```python
from build123d import *

# Parameters (mm, degrees)
SALIENTE_EXTRUIR1_DEPTH = 3
CORTAR_EXTRUIR1_DEPTH   = 10


with BuildPart() as part:
    # Croquis1 → Saliente-Extruir1 (new body)
    with BuildSketch(Plane(origin=(0, 0, 0), x_dir=(1, 0, 0), z_dir=(0, 1, 0))):
        Polygon((3, 35.5), (0, 35.5), (0, 47.5), (3, 47.5), (3, 59.5), (0, 59.5), (0, 71.5), (3, 71.5), (3, 80), (13.5, 80), (13.5, 83), (47.5, 83), (47.5, 80), (61, 80), (61, 71.5), (58, 71.5), (58, 59.5), (61, 59.5), (61, 47.5), (58, 47.5), (58, 35.5), (61, 35.5), (61, 23.5), (58, 23.5), (58, 11.5), (61, 11.5), (61, 3), (47.5, 3), (47.5, 0), (13.5, 0), (13.5, 3), (3, 3), (3, 11.5), (0, 11.5), (0, 23.5), (3, 23.5), align=None)
    extrude(amount=SALIENTE_EXTRUIR1_DEPTH)

    # Croquis2 → Cortar-Extruir1 (cut)
    with BuildSketch(Plane(origin=(0, 3, 0), x_dir=(1, 0, 0), z_dir=(0, 1, 0))):
        Polygon((15.5, 41.5), (15.5, 45.5), (12.5, 45.5), (12.5, 37.5), (15.5, 37.5), align=None)
        Polygon((45.5, 37.5), (45.5, 41.5), (45.5, 45.5), (48.5, 45.5), (48.5, 37.5), align=None)
        Polygon((30.5, 14), (23, 14), (23, 11), (25, 11), (38, 11), (38, 14), align=None)
        Polygon((35.5, 8.5), (35.5, 2.5), (38.5, 2.5), (38.5, 5.5), (38.5, 8.5), align=None)
        Polygon((22.5, 5.5), (22.5, 8.5), (25.5, 8.5), (25.5, 2.5), (22.5, 2.5), align=None)
    extrude(amount=-CORTAR_EXTRUIR1_DEPTH, mode=Mode.SUBTRACT)


solid = part.part
```
Geometry check sheet. Reference: the model listing, model coordinates, mm. A direction names the side the tool comes from. Give positions to 0.01 mm unless a question says otherwise; leave off trailing zeros. Write each loop counter-clockwise with the first axis right and the second up, starting at its lowest first coordinate (ties: lowest second). Pieces come first, ordered by that corner, then holes.
1) Section check A-A, the plane x = 30.5. Record the boundary of the cut face in (y, z), and give its area (3 significant figures).
2) Access from +Z, -Z, +X, -X, +Y, -Y to the whole of each face (thin tool, end or side, straight path). Record for faces 1 (the flat face through (60, 1, -47.5)), 2 (the flat face through (22.5, 2, -6)), 3 (the flat face through (3, 1, -29)).
3) Section check D-D, the plane x = 4.5. Record the boundary of the cut face in (y, z), and give its area (3 significant figures).
4) Release check for a two-part mould opening along Z. For faces 4 (the flat face through (2, 1, -59.5)), 5 (the flat face through (13.5, 1, -81)) record: pulls with the +Z half, pulls with the -Z half, needs draft (parallel to the pull), parting line crosses it, or undercut.
5) Gauge pin test, flat ends, axial feed: pin 1 (0.9 mm diameter, centred on x = 6, y = 2, fed in from -Z); pin 2 (0.9 mm diameter, centred on y = 2, z = -40.5, fed in from +X); pin 3 (1.5 mm diameter, centred on x = 1, y = 2, fed in from +Z). Record the tip position at first contact, or that the pin passes through.
6) Section check C-C, the plane z = -58. Record the boundary of the cut face in (x, y).
7) Section check B-B, the plane y = 0.5. State how many separate pieces and enclosed holes the cut face has, and give its area (3 significant figures).
8) Material ranges on L1, parallel to Z at x = 32.5, y = 0.3; L2, parallel to Z at x = 15, y = 0.45; L3, parallel to X at y = 1.7, z = -65, recorded low to high.
Computed:
1. outline: (0, -83) - (3, -83) - (3, -14) - (0, -14) - close; (0, -11) - (3, -11) - (3, 0) - (0, 0) - close
1. area: 240 mm2
2. face 1: +X, +Y, -Y
2. face 2: +Y, -Y
2. face 3: -X, +Y, -Y
3. outline: (0, -80) - (3, -80) - (3, -3) - (0, -3) - close
3. area: 231 mm2
4. face 4: undercut
4. face 5: needs draft
5. pin 1: stops at z = -80
5. pin 2: stops at x = 58
5. pin 3: stops at z = -11.5
6. outline: (3, 0) - (61, 0) - (61, 3) - (3, 3) - close
7. separate pieces: 1
7. enclosed holes: 5
7. area: 4,540 mm2
8. L1: z = -83 to -14, -11 to 0
8. L2: z = -83 to -45.5, -37.5 to 0
8. L3: x = 0 to 58
